from build123d import *

# Parameters (mm, degrees)
SKETCH1_W           = 47
SKETCH1_H           = 47
BOSS_EXTRUDE1_DEPTH = 10
SKETCH2_W           = 9
SKETCH2_H           = 9
CUT_EXTRUDE1_DEPTH  = 4
CUT_EXTRUDE3_DEPTH  = 53.328290628
SKETCH8_R           = 1
CUT_EXTRUDE4_DEPTH  = 68.216069507


with BuildPart() as part:
    # Sketch1 → Boss-Extrude1 (new body)
    with BuildSketch(Plane(origin=(0, 0, 0), x_dir=(1, 0, 0), z_dir=(0, 1, 0))):
        with Locations((23.5, -23.5)):
            Rectangle(SKETCH1_W, SKETCH1_H)
    extrude(amount=BOSS_EXTRUDE1_DEPTH)

    # Sketch2 → Cut-Extrude1 (cut)
    with BuildSketch(Plane(origin=(0, 0, 0), x_dir=(-1, 0, 0), z_dir=(0, -1, 0))):
        with Locations((-23.5, -23.5)):
            Rectangle(SKETCH2_W, SKETCH2_H)
    extrude(amount=-CUT_EXTRUDE1_DEPTH, mode=Mode.SUBTRACT)

    # 3DSketch1 → Cut-Extrude3 (cut, through all)
    with BuildSketch(Plane(origin=(36, 4, 9.5), x_dir=(-0.4886033689318435, 0, 0.87250601594972), z_dir=(0, -1, 0))):
        Polygon((0, 0), (12.215084223, 21.812650399), (32.718975598, 10.330471229), (20.503891375, -11.48217917), align=None)
        Polygon((22.458304851, -7.992155106), (30.764562122, 6.840447165), (42.979646346, 0), (34.673389074, -14.832602271), align=None)
    extrude(amount=-CUT_EXTRUDE3_DEPTH, mode=Mode.SUBTRACT)

    # Sketch8 → Cut-Extrude4 (cut, through all)
    with BuildSketch(Plane.XZ):
        with Locations(Location((42, 5, 0), (0, 0, 270))):
            Circle(SKETCH8_R)
        with Locations(Location((5, 5, 0), (0, 0, 270))):
            Circle(SKETCH8_R)
        with Locations(Location((5, 42, 0), (0, 0, 270))):
            Circle(SKETCH8_R)
        with Locations(Location((42, 42, 0), (0, 0, 270))):
            Circle(SKETCH8_R)
    extrude(amount=-CUT_EXTRUDE4_DEPTH, mode=Mode.SUBTRACT)


solid = part.part
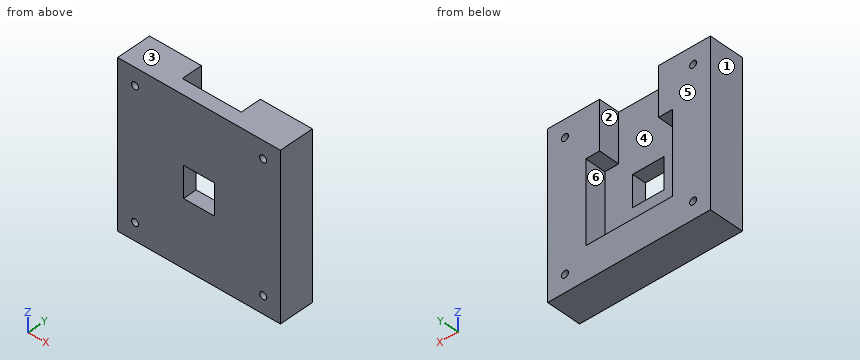
Input: part model. Units: mm. Frame: model coordinates. Face numbers are marked on the shaded views. A direction names the side the tool comes from. Coordinates: 2 decimals unless noted, no trailing zeros. Order: outer loops, then holes, each group sorted by start corner. A loop starts at its lowest first (then second) coordinate and runs counter-clockwise, first axis right, second up. Notation, with made-up numbers: M 59.5,38 L 91.5,38 A13 cw 91.5,46 Z; hole C -31,77.25 d1. An arc over 180 degrees is marked long. Write item = value, one per line. Start each with the question number.
(1) Pull-direction query (Z, two-part tool) for the marked faces 3, 4, 5 and 6; classes: released by +Z, released by -Z, zero draft, split by the parting line, or undercut.
(2) Section D-D on z = 11. Output: boundary loops of the cut face in (x, y).
(3) Reachability of the marked faces 1 and 2 from +Z, -Z, +X, -X, +Y, -Y: full face, straight path, thin tool, end or side. Return the list, or none.
(4) First-contact query: P1, Ø1.6, axis at x = 5, z = 5, coming from the -Y side (1 decimal); P2, Ø12.5, axis at x = 23, z = 30.5, coming from the +Y side; P3, Ø1.8, axis at x = 25.5, y = 6, coming from the +Z side. Flat tips, straight axial feed; report the tip coordinate or a pass-through.
(5) Line query: line 1 along X through (y, z) = (4, 5); line 2 along X through (y, z) = (3.75, 22.5); line 3 along X through (y, z) = (5.5, 42). Output: solid intervals per line, ascending. Write a range as [from, to].
(6) Section C-C on y = 6.25. Output: boundary loops of the cut face in (x, z), and give its area (3 significant figures).
(7) Section A-A on x = 42. Output: boundary loops of the cut face in (y, z), and give its area (3 significant figures).
(8) Section B-B on z = 5. Output: boundary loops of the cut face in (x, y).
Result set:
q1.face_3 = released by +Z
q1.face_4 = undercut
q1.face_5 = zero draft
q1.face_6 = undercut
q2.outline = M 0,0 L 47,0 L 47,10 L 36,10 L 36,4 L 11,4 L 11,10 L 0,10 Z
q3.face_1 = +Z, -Z, -X, +Y, -Y
q3.face_2 = +Z, +Y
q4.P1 = through
q4.P2 = 4
q4.P3 = 9.5
q5.line_1 = [0, 4], [6, 41], [43, 47]
q5.line_2 = [0, 19], [28, 47]
q5.line_3 = [0, 4], [6, 15], [32, 41], [43, 47]
q6.outline = M 0,0 L 47,0 L 47,47 L 32,47 L 32,33 L 36,33 L 36,9.5 L 11,9.5 L 11,33 L 15,33 L 15,47 L 0,47 Z; hole C 5,5 d2; hole C 5,42 d2; hole C 42,5 d2; hole C 42,42 d2
q6.area = 1,370 mm²
q7.outline = M 0,0 L 10,0 L 10,4 L 0,4 Z; M 0,6 L 10,6 L 10,41 L 0,41 Z; M 0,43 L 10,43 L 10,47 L 0,47 Z
q7.area = 430 mm²
q8.outline = M 0,0 L 4,0 L 4,10 L 0,10 Z; M 6,0 L 41,0 L 41,10 L 6,10 Z; M 43,0 L 47,0 L 47,10 L 43,10 Z
